from build123d import *

# Parameters (mm, degrees)
F0_R     = 4.25
F0_R_2   = 57
F1_DEPTH = 8


# Not quite as in the source:
# - a feature names something its author has since deleted; it is built from what else it names


with BuildPart() as f1:
    # F0 (on Front) → F1 (new body)
    with BuildSketch(Plane.XZ):
        with BuildLine():
            Line((86, -45.5504168361), (86, 0))
            ThreePointArc((86, 0), (25.52491441, -82.1247754601), (-70.8483428922, -48.7494852222))
            Line((-70.8483428922, -48.7494852222), (-52.9901534319, -77.9586575178))
            Line((-52.9901534319, -77.9586575178), (-47.1157296051, -74.3670948194))
            Line((-47.1157296051, -74.3670948194), (59.817007023, -249.2681806857))
            Line((59.817007023, -249.2681806857), (53.9425831962, -252.8597433842))
            Line((53.9425831962, -252.8597433842), (87.570656583, -307.862418303))
            ThreePointArc((87.570656583, -307.862418303), (86.7439526122, -299.1221062681), (93.1304247757, -293.0980322955))
            ThreePointArc((93.1304247757, -293.0980322955), (102.0303203377, -294.5926190657), (106.1024168691, -302.646187248))
            ThreePointArc((106.1024168691, -302.646187248), (106.1023341619, -302.6868583365), (106.1020860416, -302.7275287523))
            ThreePointArc((106.1020860416, -302.7275287523), (133.8669990345, -253.7041794438), (184.9928569387, -230.0329770139))
            ThreePointArc((184.9928569387, -230.0329770139), (176.9929095406, -222.0039661985), (185.0508781881, -214.0331874208))
            Line((185.0508781881, -214.0331874208), (108.5283892756, -203.5204235365))
            ThreePointArc((108.5283892756, -203.5204235365), (63.9114156279, -147.6449683437), (68.1014852993, -76.2644097396))
            ThreePointArc((68.1014852993, -76.2644097396), (70.6109477759, -71.1161938658), (73.4114917534, -66.1203473875))
            ThreePointArc((73.4114917534, -66.1203473875), (78.1822601822, -58.8864182021), (83.5623402825, -52.0934290975))
            ThreePointArc((83.5623402825, -52.0934290975), (85.3707897966, -49.0415912213), (86, -45.5504168361))
        make_face()
        with BuildLine():
            ThreePointArc((116.5832400171, -226.0398806244), (120.1187739231, -227.5043467184), (121.5832400171, -231.0398806244))
            ThreePointArc((121.5832400171, -231.0398806244), (113.0477061112, -234.5754145303), (116.5832400171, -226.0398806244))
        make_face(mode=Mode.SUBTRACT)
        with BuildLine():
            ThreePointArc((93.1304247757, -293.0980322955), (86.7439526122, -299.1221062681), (87.570656583, -307.862418303))
            ThreePointArc((87.570656583, -307.862418303), (98.7727093249, -312.2830715059), (106.1020860416, -302.7275287523))
            ThreePointArc((106.1020860416, -302.7275287523), (106.1023341619, -302.6868583365), (106.1024168691, -302.646187248))
            ThreePointArc((106.1024168691, -302.646187248), (102.0303203377, -294.5926190657), (93.1304247757, -293.0980322955))
        make_face()
        with BuildLine():
            ThreePointArc((100.3524168691, -302.646187248), (93.583057895, -306.0689537255), (94.8393202294, -298.5882213932))
            ThreePointArc((94.8393202294, -298.5882213932), (98.6217758433, -299.2234207705), (100.3524168691, -302.646187248))
        make_face(mode=Mode.SUBTRACT)
        with BuildLine():
            ThreePointArc((192.9928569387, -222.0329770139), (190.6701877373, -216.3966737039), (185.0508781881, -214.0331874208))
            ThreePointArc((185.0508781881, -214.0331874208), (176.9929095406, -222.0039661985), (184.9928569387, -230.0329770139))
            ThreePointArc((184.9928569387, -230.0329770139), (190.6497111882, -227.6898312634), (192.9928569387, -222.0329770139))
        make_face()
        with Locations((184.9928569387, -222.0329770139)):
            Circle(F0_R, mode=Mode.SUBTRACT)
        with BuildLine():
            ThreePointArc((-70.8483428922, -48.7494852222), (25.52491441, -82.1247754601), (86, 0))
            ThreePointArc((86, 0), (-21.0609353072, 83.3812749002), (-75.6845814881, -40.8392473605))
            Line((-75.6845814881, -40.8392473605), (-70.8483428922, -48.7494852222))
        make_face()
        with BuildLine():
            ThreePointArc((40.3259134511, 60.8508069325), (64.3148182067, 34.5341013932), (73, 0))
            ThreePointArc((73, 0), (64.3148182067, -34.5341013932), (40.3259134511, -60.8508069325))
            ThreePointArc((40.3259134511, -60.8508069325), (40.8281988477, -61.9883128671), (41, -63.2198544763))
            ThreePointArc((41, -63.2198544763), (37.5975531045, -67.5839554355), (32.5353879188, -65.3486689457))
            ThreePointArc((32.5353879188, -65.3486689457), (0, -73), (-32.5353879188, -65.3486689457))
            ThreePointArc((-32.5353879188, -65.3486689457), (-38.75, -67.1169687933), (-40.3259134511, -60.8508069325))
            ThreePointArc((-40.3259134511, -60.8508069325), (-73, 0), (-40.3259134511, 60.8508069325))
            ThreePointArc((-40.3259134511, 60.8508069325), (-38.75, 67.1169687933), (-32.5353879188, 65.3486689457))
            ThreePointArc((-32.5353879188, 65.3486689457), (0, 73), (32.5353879188, 65.3486689457))
            ThreePointArc((32.5353879188, 65.3486689457), (37.5975531045, 67.5839554355), (41, 63.2198544763))
            ThreePointArc((41, 63.2198544763), (40.8281988477, 61.9883128671), (40.3259134511, 60.8508069325))
        make_face(mode=Mode.SUBTRACT)
        with BuildLine():
            ThreePointArc((40.3259134511, -60.8508069325), (64.3148182067, -34.5341013932), (73, 0))
            ThreePointArc((73, 0), (64.3148182067, 34.5341013932), (40.3259134511, 60.8508069325))
            ThreePointArc((40.3259134511, 60.8508069325), (34.25, 59.3227401592), (32.5353879188, 65.3486689457))
            ThreePointArc((32.5353879188, 65.3486689457), (0, 73), (-32.5353879188, 65.3486689457))
            ThreePointArc((-32.5353879188, 65.3486689457), (-32.1358990407, 64.3174075808), (-32, 63.2198544763))
            ThreePointArc((-32, 63.2198544763), (-35.2684583909, 58.8916556286), (-40.3259134511, 60.8508069325))
            ThreePointArc((-40.3259134511, 60.8508069325), (-73, 0), (-40.3259134511, -60.8508069325))
            ThreePointArc((-40.3259134511, -60.8508069325), (-35.2684583909, -58.8916556286), (-32, -63.2198544763))
            ThreePointArc((-32, -63.2198544763), (-32.1358990407, -64.3174075808), (-32.5353879188, -65.3486689457))
            ThreePointArc((-32.5353879188, -65.3486689457), (0, -73), (32.5353879188, -65.3486689457))
            ThreePointArc((32.5353879188, -65.3486689457), (34.25, -59.3227401592), (40.3259134511, -60.8508069325))
        make_face()
        Circle(F0_R_2, mode=Mode.SUBTRACT)
    extrude(amount=F1_DEPTH)


solid = f1.part
The model under review builds one solid part; all positions refer to its coordinate system, in mm. A direction names the side the tool comes from. Give positions to 0.01 mm unless a question says otherwise; leave off trailing zeros. Order: outer loops, then holes, each group sorted by start corner. A loop starts at its lowest first (then second) coordinate and runs counter-clockwise, first axis right, second up. Notation, with made-up numbers: M -5,0.25 L 44,0.25 A16 cw 44,18.25 Z; hole C 68.5,59.5 d2. An arc over 180 degrees is marked long. Answer in a Markdown table with one row per item. Add a question column.
1. Mouldability with a two-part tool opening along X and no side actions: class faces 1 (the cylindrical face through (181.86, -3.94, -219.16)), 2 (the cylindrical face through (133.28, -3.94, -254.25)), 3 (the flat face through (43, -8, -98)) as released by +X, released by -X, zero draft, split by the parting line, or undercut.
2. Add section B-B on y = -2. Count the separate pieces of the cut face and the enclosed holes in it, plus the area to 3 significant figures.
3. Add section C-C on z = 17. State the section outline as (x, y) points.
4. Add section D-D on z = -193. State the section outline as (x, y) points, plus the area to 3 significant figures.
5. For pin 1 Ø2.5 at (y, z) = (-4.5, -14) entering from +X; pin 2 Ø4 at (y, z) = (-3.5, -256) entering from -X; pin 3 Ø1 at (y, z) = (-4.5, -5) entering from -X, all flat-tipped, find the tip position at first contact; note any pin that passes through.
6. Add section A-A on x = 0. State the section outline as (y, z) points.
7. To check wall thickness, follow line 1 along X through (y, z) = (-5.5, 61); line 2 along Z through (x, y) = (113.5, -2.5); line 3 along X through (y, z) = (-7, -222.5). State the ranges of each line that lie inside material, in increasing order.
8. Machinability: for faces 4 (the cylindrical face through (98.6, -3.94, -312.33)), 5 (the flat face through (86, -4, -23)), which of the approach directions +Z, -Z, +X, -X, +Y, -Y give a long, thin tool a straight path to every point of the face, cutting with its end or side? Answer none if there is none.
The answers:
| question | item | result |
|---|---|---|
| 1 | face 1 | undercut |
| 1 | face 2 | released by +X |
| 1 | face 3 | zero draft |
| 2 | separate pieces | 1 |
| 2 | enclosed holes | 8 |
| 2 | area | 31,000 mm2 |
| 3 | outline | M -84.3,-8 L -54.41,-8 L -54.41,0 L -84.3,0 Z; M 54.41,-8 L 84.3,-8 L 84.3,0 L 54.41,0 Z |
| 4 | outline | M 25.42,-8 L 93.83,-8 L 93.83,0 L 25.42,0 Z |
| 4 | area | 547 mm2 |
| 5 | pin 1 | x = 86 |
| 5 | pin 2 | x = 54.64 |
| 5 | pin 3 | x = -85.88 |
| 6 | outline | M -8,-151.43 L 0,-151.43 L 0,-57 L -8,-57 Z; M -8,57 L 0,57 L 0,86 L -8,86 Z |
| 7 | line 1 | -60.62 to -40.41, -32.59 to 32.59, 40.41 to 60.62 |
| 7 | line 2 | -281.06 to -234.98, -227.1 to -204.2 |
| 7 | line 3 | 43.45 to 180.77, 189.22 to 192.98 |
| 8 | face 4 | -Z, +Y, -Y |
| 8 | face 5 | +Z, +X, +Y, -Y |
